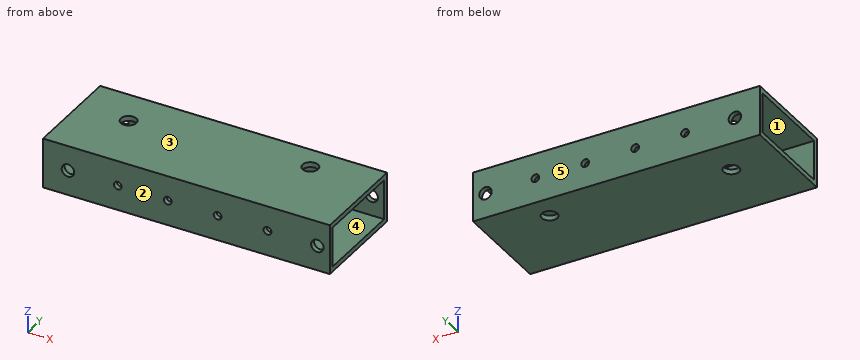
Autodesk Inventor part; units mm, degrees
ref_plane "YZ Plane" through (0, 0, 0) normal (1, 0, 0) x (0, 1, 0)
ref_plane "XZ Plane" through (0, 0, 0) normal (0, 1, 0) x (-1, 0, 0)
ref_plane "XY Plane" through (0, 0, 0) normal (0, 0, 1) x (1, 0, 0)
sketch "Sketch1" plane through (0, 0, 0) normal (1, 0, 0) x (0, 1, 0)
  line L0 (0, 0) -> (50.8, 0)
  line L1 (50.8, 0) -> (50.8, -25.4)
  line L2 (50.8, -25.4) -> (0, -25.4)
  line L3 (0, -25.4) -> (0, 0)
  line L4 (2.54, -2.54) -> (48.26, -2.54)
  line L5 (48.26, -2.54) -> (48.26, -22.86)
  line L6 (48.26, -22.86) -> (2.54, -22.86)
  line L7 (2.54, -22.86) -> (2.54, -2.54)
  dimension "d0" = 50.8
  dimension "d1" = 25.4
  dimension "d2" = 45.72
  dimension "d3" = 20.32
  dimension "d4" = 2.54
  dimension "d5" = 2.54
extrude "Extrusion1" add sketch "Sketch1" along normal blind 146.05
sketch "Sketch5" plane through (0, 50.8, 0) normal (0, 1, 0) x (1, 0, 0)
  line L0 (0, 0) -> (0, 25.4)
  line L1 (0, 0) -> (146.05, 0)
  line L2 (146.05, 25.4) -> (146.05, 0)
  line L3 (0, 25.4) -> (146.05, 25.4)
  point P0 (12.7, 12.7)
  dimension "d39" = 12.7
  dimension "d40" = 12.7
hole "Hole3" at (12.7, 50.8, -12.7) direction (0, -1, 0) diameter 3.9688 end through all
pattern_linear "Rectangular Pattern1" count 6 spacing 25.4 along (1, 0, 0) of "Hole3"
sketch "Sketch6" plane through (0, 0, -25.4) normal (0, 0, -1) x (-1, 0, 0)
  line L0 (0, 50.8) -> (0, 0)
  line L1 (0, 50.8) -> (-146.05, 50.8)
  line L2 (-146.05, 0) -> (-146.05, 50.8)
  line L3 (0, 0) -> (-146.05, 0)
  point P0 (-114.3, 38.1)
  dimension "d51" = 12.7
  dimension "d52" = 31.75
hole "Hole4" at (114.3, 38.1, -25.4) direction (0, 0, 1) diameter 7.9375 end through all
sketch "Sketch7" plane through (0, 50.8, 0) normal (0, 1, 0) x (1, 0, 0)
  circle A0 centre (139.7, 12.7) radius 1.9844
  circle A1 centre (114.3, 12.7) radius 1.9844
  circle A2 centre (88.9, 12.7) radius 1.9844
  circle A3 centre (63.5, 12.7) radius 1.9844
  circle A4 centre (38.1, 12.7) radius 1.9844
  circle A5 centre (12.7, 12.7) radius 1.9844
  line L0 (0, 0) -> (0, 25.4)
  line L1 (0, 0) -> (146.05, 0)
  line L2 (146.05, 25.4) -> (146.05, 0)
  line L3 (0, 25.4) -> (146.05, 25.4)
  circle A6 centre (12.7, 12.7) radius 1.9844
  circle A7 centre (12.7, 12.7) radius 3.175
  circle A8 centre (139.7, 12.7) radius 3.175
  dimension "d60" = 6.35
  dimension "d61" = 6.35
extrude "Extrusion3" cut sketch "Sketch7" against normal blind 50.8 contours A7 | A8
sketch "Sketch8" plane through (0, 0, -25.4) normal (0, 0, -1) x (-1, 0, 0)
  circle A0 centre (-114.3, 38.1) radius 3.9687
  line L0 (0, 50.8) -> (0, 0)
  line L1 (0, 50.8) -> (-146.05, 50.8)
  line L2 (-146.05, 0) -> (-146.05, 50.8)
  line L3 (0, 0) -> (-146.05, 0)
  point P0 (-25.4, 31.75)
  dimension "d64" = 19.05
  dimension "d65" = 25.4
hole "Hole5" at (25.4, 31.75, -25.4) direction (0, 0, 1) diameter 7.9375 end through all
properties part number "frame_front_bumper"
Geometry: final body of the model. Coordinates: model frame, mm. Face numbers are marked on the shaded views. A direction names the side the tool comes from. Round coordinates to 2 decimals unless told otherwise and drop trailing zeros. Write each loop counter-clockwise with the first axis right and the second up, starting at its lowest first coordinate (ties: lowest second). Pieces come first, ordered by that corner, then holes. Notation, with made-up numbers: (-6, 46.5) -> (32, 46.5) arc R20 ccw to (32, 72.5) -> close; hole circle Ø7 at (83, -12). An arc over 180 degrees is marked (long way). Return JSON: item names as keys, results as strings.
Q1. Section C-C on y = 31.75. Return the cut outline in (x, z), and give its area (3 significant figures).
From the geometry:
{"outline": "(0, -25.4) -> (21.43, -25.4) -> (21.43, -22.86) -> (0, -22.86) -> close; (0, -2.54) -> (21.43, -2.54) -> (21.43, 0) -> (0, 0) -> close; (29.37, -25.4) -> (146.05, -25.4) -> (146.05, -22.86) -> (29.37, -22.86) -> close; (29.37, -2.54) -> (146.05, -2.54) -> (146.05, 0) -> (29.37, 0) -> close", "area": "702 mm2"}
Q2. Set-up query: the marked faces 1 and 2. Return all of +Z, -Z, +X, -X, +Y, -Y with unobstructed straight access to the full face (end or side cutting, diameter ignored); none if empty.
From the geometry:
{"face 1": "+X, -X", "face 2": "+Z, -Z, +X, -X, -Y"}
Q3. First-contact query: pin 1 Ø6.5 at (x, z) = (38.1, -12.7) entering from -Y; pin 2 Ø12 at (y, z) = (41, -14.5) entering from -X (1 decimal). Flat tips, straight axial feed; report the tip coordinate or a pass-through.
From the geometry:
{"pin 1": "y = 0", "pin 2": "through"}
Q4. Mould query, pull axis Z, two halves, no side actions, for the marked faces 3, 4 and 5. Classes: +Z half, -Z half, draft (parallel to the pull), parting line (faces both ways), or undercut.
From the geometry:
{"face 3": "+Z half", "face 4": "undercut", "face 5": "draft"}
Q5. Section D-D on x = 12.7. Return the cut outline in (y, z) (3 decimals), and give its area (3 significant figures).
From the geometry:
{"outline": "(0, -25.4) -> (50.8, -25.4) -> (50.8, -15.875) -> (48.26, -15.875) -> (48.26, -22.86) -> (2.54, -22.86) -> (2.54, -15.875) -> (0, -15.875) -> close; (0, -9.525) -> (2.54, -9.525) -> (2.54, -2.54) -> (48.26, -2.54) -> (48.26, -9.525) -> (50.8, -9.525) -> (50.8, 0) -> (0, 0) -> close", "area": "329 mm2"}
Q6. Section B-B on z = -17.5. Return the cut outline in (x, y).
From the geometry:
{"outline": "(0, 0) -> (146.05, 0) -> (146.05, 2.54) -> (0, 2.54) -> close; (0, 48.26) -> (146.05, 48.26) -> (146.05, 50.8) -> (0, 50.8) -> close"}
Q7. Section A-A on y = 12.5. Return the cut outline in (x, z).
From the geometry:
{"outline": "(0, -25.4) -> (146.05, -25.4) -> (146.05, -22.86) -> (0, -22.86) -> close; (0, -2.54) -> (146.05, -2.54) -> (146.05, 0) -> (0, 0) -> close"}
Q8. Ray query, line 1 (Z direction, x = 57, y = 3); line 2 (Y direction, x = 49, z = -16.75); line 3 (Z direction, x = 12.7, y = 49.2) (3 decimals). Return the intervals inside material, ascending.
From the geometry:
{"line 1": "-25.4 to -22.86, -2.54 to 0", "line 2": "0 to 2.54, 48.26 to 50.8", "line 3": "-25.4 to -15.875, -9.525 to 0"}
